Geometry check sheet. Reference: the model listing, model coordinates, mm. Face numbers are marked on the shaded views. A direction names the side the tool comes from. Give positions to 0.01 mm unless a question says otherwise; leave off trailing zeros. Order: outer loops, then holes, each group sorted by start corner. A loop starts at its lowest first (then second) coordinate and runs counter-clockwise, first axis right, second up. Notation, with made-up numbers: M -22,73 L 3,73 A16 ccw 3,95 Z; hole C 76,54.5 d3. An arc over 180 degrees is marked long. Answer as CSV lines item,"result". Start each with the question number.
Q1. Section check C-C, the plane x = 17. Record the boundary of the cut face in (y, z).
Q2. Mould release check, pull along X, two halves, no side actions. Record for the marked faces 1, 2, 3 and 4: +X half, -X half, draft (parallel to the pull), parting line (faces both ways), or undercut.
Q3. Section check B-B, the plane y = 2.5. Record the boundary of the cut face in (x, z) (3 decimals).
Q4. Go/stop test with flat-tipped pins: pin 1 (12 mm diameter, centred on x = 2, y = 18, fed in from -Z); pin 2 (1 mm diameter, centred on x = -31.5, y = -7.5, fed in from -Z). Record where each tip stops, or that it passes through.
Q5. Section check A-A, the plane z = -9.25. Record the boundary of the cut face in (x, y), then the cut area to 3 significant figures.
Q6. Section check D-D, the plane z = -4.25. Record the boundary of the cut face in (x, y).
Q7. Thickness scan on line 1 (X direction, y = 20, z = -9.5); line 2 (X direction, y = -18.5, z = -14); line 3 (X direction, y = -19.5, z = -5.5). Record the ranges inside material, lowest first.
Q8. Set-up check for the marked faces 5 and 6: record each of +Z, -Z, +X, -X, +Y, -Y from which the full face is reachable in a straight line by a thin tool's end or side.
```python
from build123d import *

# Parameters (mm, degrees)
F0_W          = 88
F0_H          = 46.4
F1_DEPTH      = 17.65
F2_W          = 50
F2_H          = 46.4
F3_DEPTH      = 6.15
F5_DEPTH      = 23.201
F5_DEPTH_BACK = 23.201


with BuildPart() as f1:
    # F0 (on Top) → F1 (new body)
    with BuildSketch(Plane.XY):
        Rectangle(F0_W, F0_H)
    extrude(amount=-F1_DEPTH)

    # F2 (on face) → F3 (cut)
    with BuildSketch(Plane(origin=(0, 0, -17.65), x_dir=(1, 0, 0), z_dir=(0, 0, -1))):
        Rectangle(F2_W, F2_H)
    extrude(amount=-F3_DEPTH, mode=Mode.SUBTRACT)

    # F4 (on Front) → F5 (cut, two sides)
    with BuildSketch(Plane.XZ) as f5_sk:
        with BuildLine():
            Line((-40, -7.95), (-40, -17.65))
            Line((-40, -17.65), (-28.41, -17.65))
            Line((-28.41, -17.65), (-28.41, -7.95))
            ThreePointArc((-28.41, -7.95), (-34.205, -2.155), (-40, -7.95))
        make_face()
        with BuildLine():
            Line((28.21, -7.95), (28.21, -17.65))
            Line((28.21, -17.65), (39.8, -17.65))
            Line((39.8, -17.65), (39.8, -7.95))
            ThreePointArc((39.8, -7.95), (34.005, -2.155), (28.21, -7.95))
        make_face()
    extrude(amount=-F5_DEPTH, mode=Mode.SUBTRACT)
    extrude(f5_sk.sketch, amount=F5_DEPTH_BACK, mode=Mode.SUBTRACT)


solid = f1.part
```
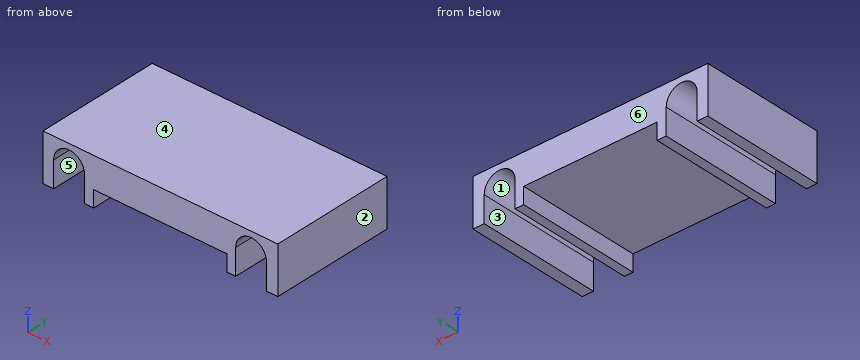
Answer block:
1,outline,"M -23.2,-11.5 L 23.2,-11.5 L 23.2,0 L -23.2,0 Z"
2,face 1,"undercut"
2,face 2,"+X half"
2,face 3,"undercut"
2,face 4,"draft"
3,outline,"M -44,-17.65 L -40,-17.65 L -40,-7.95 A5.795 cw -28.41,-7.95 L -28.41,-17.65 L -25,-17.65 L -25,-11.5 L 25,-11.5 L 25,-17.65 L 28.21,-17.65 L 28.21,-7.95 A5.795 cw 39.8,-7.95 L 39.8,-17.65 L 44,-17.65 L 44,0 L -44,0 Z"
4,pin 1,"stops at z = -11.5"
4,pin 2,"stops at z = -3.12"
5,outline,"M -44,-23.2 L -40,-23.2 L -40,23.2 L -44,23.2 Z; M -28.41,-23.2 L 28.21,-23.2 L 28.21,23.2 L -28.41,23.2 Z; M 39.8,-23.2 L 44,-23.2 L 44,23.2 L 39.8,23.2 Z"
5,area,"3,010 mm2"
6,outline,"M -44,-23.2 L -38.67,-23.2 L -38.67,23.2 L -44,23.2 Z; M -29.74,-23.2 L 29.54,-23.2 L 29.54,23.2 L -29.74,23.2 Z; M 38.47,-23.2 L 44,-23.2 L 44,23.2 L 38.47,23.2 Z"
7,line 1,"x = -44 to -40, -28.41 to 28.21, 39.8 to 44"
7,line 2,"x = -44 to -40, -28.41 to -25, 25 to 28.21, 39.8 to 44"
7,line 3,"x = -44 to -39.46, -28.95 to 28.75, 39.26 to 44"
8,face 5,"-Z, +Y, -Y"
8,face 6,"+Z, -Z, +X, -X, +Y"
